Input: part model. Units: mm. Frame: model coordinates. Face numbers are marked on the shaded views. Coordinates: 2 decimals unless noted, no trailing zeros. Write each loop counter-clockwise with the first axis right and the second up, starting at its lowest first coordinate (ties: lowest second). Pieces come first, ordered by that corner, then holes. Notation, with made-up numbers: M -23,12 L -9,12 A32 ccw -9,48 Z; hole C 37,50.25 d7. An arc over 180 degrees is marked long. Answer as a JSON object with one key per item and string values. Group by question number.
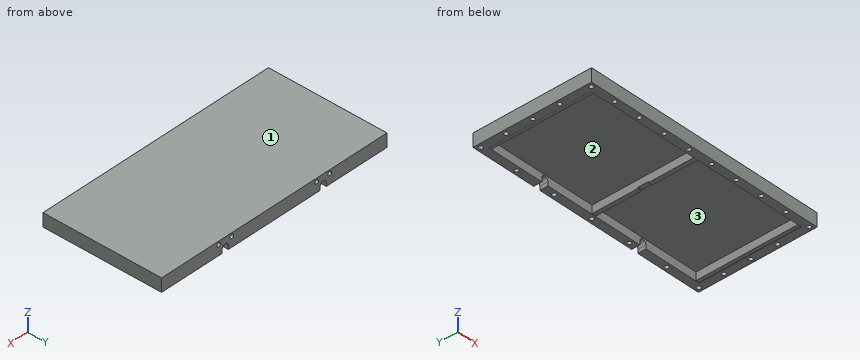
from build123d import *

# Parameters (mm, degrees)
F0_W      = 150
F0_H      = 73
F1_DEPTH  = 8.127
F3_R      = 1.25
F4_DEPTH  = 5
F5_R      = 1.25
F6_DEPTH  = 5
F7_R      = 1.25
F8_DEPTH  = 5
F9_R      = 1.25
F10_DEPTH = 5
F11_R     = 1.25
F12_DEPTH = 5
F13_R     = 1.25
F14_DEPTH = 5
F15_R     = 1.25
F16_DEPTH = 5
F17_R     = 1.25
F18_DEPTH = 5
F19_R     = 1.25
F20_DEPTH = 5
F21_R     = 1.25
F22_DEPTH = 5
F23_R     = 1.25
F24_DEPTH = 5
F25_R     = 1.25
F26_DEPTH = 5
F27_R     = 1.25
F28_DEPTH = 5
F29_R     = 1.25
F30_DEPTH = 5
F31_R     = 1.25
F32_DEPTH = 5
F33_R     = 1.25
F34_DEPTH = 5
F35_R     = 1.25
F36_DEPTH = 5
F37_R     = 1.25
F38_DEPTH = 5
F39_R     = 1.25
F40_DEPTH = 5
F41_R     = 1.25
F42_DEPTH = 5
F43_R     = 1.25
F44_DEPTH = 5
F45_R     = 1.25
F46_DEPTH = 5
F47_R     = 1.25
F48_DEPTH = 5
F2_W      = 136
F2_H      = 63
F49_DEPTH = 5.127
F50_W     = 2.5
F50_H     = 63
F51_DEPTH = 4.873
F52_W     = 6.5
F52_H     = 0.623
F53_DEPTH = 2.5
F54_W     = 2
F54_H     = 63
F55_DEPTH = 0.254
F56_W     = 2
F56_H     = 63
F57_DEPTH = 0.254
F58_R     = 2.05
F59_DEPTH = 5
F60_R     = 2.05
F61_DEPTH = 5
F62_W     = 4.1
F62_H     = 2.304
F63_DEPTH = 5
F64_W     = 4.1
F64_H     = 2.304
F65_DEPTH = 5
F66_R     = 1.25
F67_DEPTH = 2.5


with BuildPart() as f1:
    # F0 (on Top) → F1 (new body)
    with BuildSketch(Plane.XY):
        with Locations((75, 36.5)):
            Rectangle(F0_W, F0_H)
    extrude(amount=F1_DEPTH)

    # F3 (on face) → F4 (cut)
    with BuildSketch(Plane(origin=(0, 0, 0), x_dir=(1, 0, 0), z_dir=(0, 0, -1))):
        with Locations((2.5, -2.5)):
            Circle(F3_R)
    extrude(amount=-F4_DEPTH, mode=Mode.SUBTRACT)

    # F5 (on face) → F6 (cut)
    with BuildSketch(Plane(origin=(0, 0, 0), x_dir=(1, 0, 0), z_dir=(0, 0, -1))):
        with Locations((2.5, -22)):
            Circle(F5_R)
    extrude(amount=-F6_DEPTH, mode=Mode.SUBTRACT)

    # F7 (on face) → F8 (cut)
    with BuildSketch(Plane(origin=(0, 0, 0), x_dir=(1, 0, 0), z_dir=(0, 0, -1))):
        with Locations((147.5, -2.5)):
            Circle(F7_R)
    extrude(amount=-F8_DEPTH, mode=Mode.SUBTRACT)

    # F9 (on face) → F10 (cut)
    with BuildSketch(Plane(origin=(0, 0, 0), x_dir=(1, 0, 0), z_dir=(0, 0, -1))):
        with Locations((147.5, -22)):
            Circle(F9_R)
    extrude(amount=-F10_DEPTH, mode=Mode.SUBTRACT)

    # F11 (on face) → F12 (cut)
    with BuildSketch(Plane(origin=(0, 0, 0), x_dir=(1, 0, 0), z_dir=(0, 0, -1))):
        with Locations((2.5, -38.5)):
            Circle(F11_R)
    extrude(amount=-F12_DEPTH, mode=Mode.SUBTRACT)

    # F13 (on face) → F14 (cut)
    with BuildSketch(Plane(origin=(0, 0, 0), x_dir=(1, 0, 0), z_dir=(0, 0, -1))):
        with Locations((147.5, -38.5)):
            Circle(F13_R)
    extrude(amount=-F14_DEPTH, mode=Mode.SUBTRACT)

    # F15 (on face) → F16 (cut)
    with BuildSketch(Plane(origin=(0, 0, 0), x_dir=(1, 0, 0), z_dir=(0, 0, -1))):
        with Locations((2.5, -55)):
            Circle(F15_R)
    extrude(amount=-F16_DEPTH, mode=Mode.SUBTRACT)

    # F17 (on face) → F18 (cut)
    with BuildSketch(Plane(origin=(0, 0, 0), x_dir=(1, 0, 0), z_dir=(0, 0, -1))):
        with Locations((147.5, -55)):
            Circle(F17_R)
    extrude(amount=-F18_DEPTH, mode=Mode.SUBTRACT)

    # F19 (on face) → F20 (cut)
    with BuildSketch(Plane(origin=(0, 0, 0), x_dir=(1, 0, 0), z_dir=(0, 0, -1))):
        with Locations((2.5, -70.5)):
            Circle(F19_R)
    extrude(amount=-F20_DEPTH, mode=Mode.SUBTRACT)

    # F21 (on face) → F22 (cut)
    with BuildSketch(Plane(origin=(0, 0, 0), x_dir=(1, 0, 0), z_dir=(0, 0, -1))):
        with Locations((147.5, -70.5)):
            Circle(F21_R)
    extrude(amount=-F22_DEPTH, mode=Mode.SUBTRACT)

    # F23 (on face) → F24 (cut)
    with BuildSketch(Plane(origin=(0, 0, 0), x_dir=(1, 0, 0), z_dir=(0, 0, -1))):
        with Locations((18, -2.5)):
            Circle(F23_R)
    extrude(amount=-F24_DEPTH, mode=Mode.SUBTRACT)

    # F25 (on face) → F26 (cut)
    with BuildSketch(Plane(origin=(0, 0, 0), x_dir=(1, 0, 0), z_dir=(0, 0, -1))):
        with Locations((26.25, -70.5)):
            Circle(F25_R)
    extrude(amount=-F26_DEPTH, mode=Mode.SUBTRACT)

    # F27 (on face) → F28 (cut)
    with BuildSketch(Plane(origin=(0, 0, 0), x_dir=(1, 0, 0), z_dir=(0, 0, -1))):
        with Locations((34.5, -2.5)):
            Circle(F27_R)
    extrude(amount=-F28_DEPTH, mode=Mode.SUBTRACT)

    # F29 (on face) → F30 (cut)
    with BuildSketch(Plane(origin=(0, 0, 0), x_dir=(1, 0, 0), z_dir=(0, 0, -1))):
        with Locations((51, -2.5)):
            Circle(F29_R)
    extrude(amount=-F30_DEPTH, mode=Mode.SUBTRACT)

    # F31 (on face) → F32 (cut)
    with BuildSketch(Plane(origin=(0, 0, 0), x_dir=(1, 0, 0), z_dir=(0, 0, -1))):
        with Locations((51.25, -70.5)):
            Circle(F31_R)
    extrude(amount=-F32_DEPTH, mode=Mode.SUBTRACT)

    # F33 (on face) → F34 (cut)
    with BuildSketch(Plane(origin=(0, 0, 0), x_dir=(1, 0, 0), z_dir=(0, 0, -1))):
        with Locations((67.5, -2.5)):
            Circle(F33_R)
    extrude(amount=-F34_DEPTH, mode=Mode.SUBTRACT)

    # F35 (on face) → F36 (cut)
    with BuildSketch(Plane(origin=(0, 0, 0), x_dir=(1, 0, 0), z_dir=(0, 0, -1))):
        with Locations((76.25, -70.5)):
            Circle(F35_R)
    extrude(amount=-F36_DEPTH, mode=Mode.SUBTRACT)

    # F37 (on face) → F38 (cut)
    with BuildSketch(Plane(origin=(0, 0, 0), x_dir=(1, 0, 0), z_dir=(0, 0, -1))):
        with Locations((82.5, -2.5)):
            Circle(F37_R)
    extrude(amount=-F38_DEPTH, mode=Mode.SUBTRACT)

    # F39 (on face) → F40 (cut)
    with BuildSketch(Plane(origin=(0, 0, 0), x_dir=(1, 0, 0), z_dir=(0, 0, -1))):
        with Locations((99, -2.5)):
            Circle(F39_R)
    extrude(amount=-F40_DEPTH, mode=Mode.SUBTRACT)

    # F41 (on face) → F42 (cut)
    with BuildSketch(Plane(origin=(0, 0, 0), x_dir=(1, 0, 0), z_dir=(0, 0, -1))):
        with Locations((101.25, -70.5)):
            Circle(F41_R)
    extrude(amount=-F42_DEPTH, mode=Mode.SUBTRACT)

    # F43 (on face) → F44 (cut)
    with BuildSketch(Plane(origin=(0, 0, 0), x_dir=(1, 0, 0), z_dir=(0, 0, -1))):
        with Locations((115.5, -2.5)):
            Circle(F43_R)
    extrude(amount=-F44_DEPTH, mode=Mode.SUBTRACT)

    # F45 (on face) → F46 (cut)
    with BuildSketch(Plane(origin=(0, 0, 0), x_dir=(1, 0, 0), z_dir=(0, 0, -1))):
        with Locations((126.25, -70.5)):
            Circle(F45_R)
    extrude(amount=-F46_DEPTH, mode=Mode.SUBTRACT)

    # F47 (on face) → F48 (cut)
    with BuildSketch(Plane(origin=(0, 0, 0), x_dir=(1, 0, 0), z_dir=(0, 0, -1))):
        with Locations((132, -2.5)):
            Circle(F47_R)
    extrude(amount=-F48_DEPTH, mode=Mode.SUBTRACT)

    # F2 (on Top) → F49 (cut)
    with BuildSketch(Plane.XY):
        with Locations((75, 36.5)):
            Rectangle(F2_W, F2_H)
    extrude(amount=F49_DEPTH, mode=Mode.SUBTRACT)

    # F50 (on face) → F51 (join)
    with BuildSketch(Plane(origin=(0, 0, 5.127), x_dir=(1, 0, 0), z_dir=(0, 0, -1))):
        with Locations((75, -36.5)):
            Rectangle(F50_W, F50_H)
    extrude(amount=F51_DEPTH)

    # F52 (on face) → F53 (cut)
    with BuildSketch(Plane.YZ.offset(76.25)):
        with Locations((36.5, 0.5655)):
            Rectangle(F52_W, F52_H)
    extrude(amount=-F53_DEPTH, mode=Mode.SUBTRACT)

    # F54 (on face) → F55 (cut)
    with BuildSketch(Plane(origin=(0, 0, 0), x_dir=(1, 0, 0), z_dir=(0, 0, -1))):
        with Locations((6, -36.5)):
            Rectangle(F54_W, F54_H)
    extrude(amount=-F55_DEPTH, mode=Mode.SUBTRACT)

    # F56 (on face) → F57 (cut)
    with BuildSketch(Plane(origin=(0, 0, 0), x_dir=(1, 0, 0), z_dir=(0, 0, -1))):
        with Locations((144, -36.5)):
            Rectangle(F56_W, F56_H)
    extrude(amount=-F57_DEPTH, mode=Mode.SUBTRACT)

    # F58 (on face) → F59 (cut)
    with BuildSketch(Plane(origin=(0, 73, 0), x_dir=(-1, 0, 0), z_dir=(0, 1, 0))):
        with Locations((-42.4, 2.304)):
            Circle(F58_R)
    extrude(amount=-F59_DEPTH, mode=Mode.SUBTRACT)

    # F60 (on face) → F61 (cut)
    with BuildSketch(Plane(origin=(0, 73, 0), x_dir=(-1, 0, 0), z_dir=(0, 1, 0))):
        with Locations((-107.6, 2.304)):
            Circle(F60_R)
    extrude(amount=-F61_DEPTH, mode=Mode.SUBTRACT)

    # F62 (on face) → F63 (cut)
    with BuildSketch(Plane(origin=(0, 73, 0), x_dir=(-1, 0, 0), z_dir=(0, 1, 0))):
        with Locations((-107.6, 1.152)):
            Rectangle(F62_W, F62_H)
    extrude(amount=-F63_DEPTH, mode=Mode.SUBTRACT)

    # F64 (on face) → F65 (cut)
    with BuildSketch(Plane(origin=(0, 73, 0), x_dir=(-1, 0, 0), z_dir=(0, 1, 0))):
        with Locations((-42.4, 1.152)):
            Rectangle(F64_W, F64_H)
    extrude(amount=-F65_DEPTH, mode=Mode.SUBTRACT)

    # F66 (on face) → F67 (cut)
    with BuildSketch(Plane(origin=(0, 73, 0), x_dir=(-1, 0, 0), z_dir=(0, 1, 0))):
        with Locations((-38.1, 6.077)):
            Circle(F66_R)
        with Locations((-46.7, 6.077)):
            Circle(F66_R)
        with Locations((-111.9, 6.077)):
            Circle(F66_R)
        with Locations((-103.3, 6.077)):
            Circle(F66_R)
    extrude(amount=-F67_DEPTH, mode=Mode.SUBTRACT)


solid = f1.part
Q1. Draft query along Y for the marked faces 1, 2 and 3. Return one class per face: released by +Y, released by -Y, zero draft, split by the parting line, or undercut.
Q2. Line query: line 1 (Y direction, x = 67.5, z = 3.4); line 2 (X direction, y = 31, z = 1); line 3 (X direction, y = 38.5, z = 1). Output: solid intervals per line, ascending. Write a range as from..to.
Q3. Section B-B, the plane y = 9.5. Return the cut outline in (x, z).
Q4. Pin query (flat end, axial travel): pin 1 Ø1.2 at (x, y) = (74.5, 60.5) entering from -Z; pin 2 Ø12 at (x, y) = (121, 46) entering from -Z; pin 3 Ø0.8 at (x, y) = (3, 21.5) entering from -Z. Return the tip coordinate at first contact, or that it passes through.
Q5. Section C-C, the plane x = 42.4. Return the cut outline in (y, z), and give its area (4 significant figures).
Q6. Section A-A, the plane x = 9.5. Return the cut outline in (y, z), and give its area (3 significant figures).
Filled in:
{
 "1": {"face 1": "zero draft", "face 2": "undercut", "face 3": "undercut"},
 "2": {"line 1": "0..1.25, 3.75..5, 68..73", "line 2": "0..7, 73.75..76.25, 143..150", "line 3": "0..1.25, 3.75..7, 73.75..76.25, 143..146.25, 148.75..150"},
 "3": {"outline": "M 0,0 L 5,0 L 5,0.25 L 7,0.25 L 7,5.13 L 73.75,5.13 L 73.75,0.25 L 76.25,0.25 L 76.25,5.13 L 143,5.13 L 143,0.25 L 145,0.25 L 145,0 L 150,0 L 150,8.13 L 0,8.13 Z"},
 "4": {"pin 1": "z = 0.25", "pin 2": "z = 5.13", "pin 3": "z = 5"},
 "5": {"outline": "M 0,0 L 5,0 L 5,5.13 L 68,5.13 L 68,4.35 L 73,4.35 L 73,8.13 L 0,8.13 Z", "area": "248.5 mm^2"},
 "6": {"outline": "M 0,0 L 5,0 L 5,5.13 L 68,5.13 L 68,0 L 73,0 L 73,8.13 L 0,8.13 Z", "area": "270 mm^2"}
}
